Build history of the part. All positions in model axes, mm. A direction names the side the tool comes from. Round coordinates to 2 decimals unless told otherwise and drop trailing zeros. Write each loop counter-clockwise with the first axis right and the second up, starting at its lowest first coordinate (ties: lowest second). Pieces come first, ordered by that corner, then holes.
1) Which spindle directions (+Z, -Z, +X, -X, +Y, -Y) get a long thin tool onto all of the face, cutting with end or side? Do faces 4 (the flat face through (-8, -41, -69.596)), 5 (the cylindrical face through (-1.1, -33.14, -73.57)), 6 (the flat face through (-57.29, -28, -66)). Say none if no direction does.
2) Wall check: probe 1 along X at (y, z) = (-38.1, -51.65); probe 2 along X at (y, z) = (-29, -64); probe 3 along X at (y, z) = (-47, -63). Give the ranges that are in metal, low to high.
3) Saw through at D-D (x = -70). Write the cut outline in (y, z), plus the area to 3 significant figures.
4) Saw through at A-A (z = -73.5). Write the cut outline in (x, y) (1 decimal), plus the area to 3 significant figures.
5) Saw through at B-B (x = 30). Write the cut outline in (y, z).
6) Saw through at C-C (z = -63.5). State how many separate pieces and enclosed holes the cut face has, plus the area to 3 significant figures.
7) Flat gauge pins, fed straight in: pin 1 (12 mm diameter, centred on x = 35.5, z = -64, fed in from -Y); pin 2 (10 mm diameter, centred on y = -45, z = -72, fed in from +X); pin 3 (5 mm diameter, centred on y = -26, z = -71.5, fed in from -X); pin 4 (3 mm diameter, centred on x = 30, z = -63.5, fed in from +Y). Where does each tip first touch, or does it go through?
8) Pull direction Z, two halves, no side cores. Call faces 1 (the cylindrical face through (20.071, -17.413, -63.322)), 2 (the flat face through (67, -41, -52.2)), 3 (the flat face through (0, -46, -70.866)): +Z half, -Z half, draft (parallel to the pull), parting line (faces both ways), or undercut.
Autodesk Inventor part; units mm, degrees
ref_plane "YZ Plane" through (0, 0, 0) normal (1, 0, 0) x (0, 1, 0)
ref_plane "XZ Plane" through (0, 0, 0) normal (0, 1, 0) x (-1, 0, 0)
ref_plane "XY Plane" through (0, 0, 0) normal (0, 0, 1) x (1, 0, 0)
ref_plane "Work Plane1" through (0, 0, -76.2) normal (0, 0, 1) x (1, 0, 0)
sketch "Sketch1" plane through (0, 0, -76.2) normal (0, 0, 1) x (1, 0, 0)
  line L0 (-80, -10.16) -> (80, -10.16)
  circle A0 centre (70, -38.1) radius 4
  circle A1 centre (-70, -38.1) radius 4
  arc A2 (82.7105, -38.1) -> (57.2895, -38.1) centre (70, -38.1) ccw
  arc A3 (57.2895, -38.1) -> (82.4735, -35.6569) centre (70, -38.1) ccw
  arc A4 (-82.4735, -35.6569) -> (-57.2895, -38.1) centre (-70, -38.1) ccw
  line L1 (82.7105, -38.1) -> (80, -10.16)
  line L2 (-82.7105, -38.1) -> (-80, -10.16)
  circle A5 centre (0, -38.1) radius 5.08
  line L3 (17.78, -25.4) -> (17.78, -50.8)
  line L4 (17.78, -50.8) -> (-17.78, -50.8)
  line L5 (-17.78, -50.8) -> (-17.78, -25.4)
  line L6 (-17.78, -25.4) -> (17.78, -50.8) construction
  line L7 (17.78, -25.4) -> (-17.78, -50.8) construction
  line L8 (80, -10.16) -> (-80, -10.16)
  line L9 (-17.78, -15.24) -> (-57.2895, -15.24)
  line L10 (17.78, -15.24) -> (57.2895, -15.24)
  line L11 (57.2895, -38.1) -> (57.2895, -15.24)
  line L12 (-57.2895, -38.1) -> (-57.2895, -15.24)
  line L13 (-17.78, -38.1) -> (-17.78, -15.24)
  line L14 (17.78, -38.1) -> (17.78, -15.24)
  point P0 (0, 0)
  dimension "d0" = 10.16
  dimension "d2" = 35.56
  dimension "d3" = 25.4
extrude "Extrusion1" add sketch "Sketch1" along normal blind 25.4 contours L0 L1 A2 L11 L10 L14 L3 L4 L5 L13 L9 L12 A4 L2 | L1 A3 A2 | A2 L1
sketch "Sketch2" plane through (0, 0, -76.2) normal (0, 0, -1) x (-1, 0, 0)
  circle A0 centre (-70, -38.1) radius 4
  circle A1 centre (-70, -38.1) radius 7.5
  circle A2 centre (70, -38.1) radius 4
  circle A3 centre (70, -38.1) radius 7.5
  point P0 (0, 0)
  dimension "d7" = 15
  dimension "d8" = 15
extrude "Extrusion2" cut sketch "Sketch2" against normal blind 24
sketch "Sketch3" plane through (-17.78, -50.8, -76.2) normal (0, -1, 0) x (1, 0, 0)
  line L0 (0, 0) -> (35.56, 0)
  line L1 (0, 0) -> (0, 25.4)
  line L2 (0, 25.4) -> (35.56, 25.4)
  line L3 (35.56, 0) -> (35.56, 25.4)
  line L4 (12.7, 0) -> (12.7, 25.4)
  line L5 (22.86, 0) -> (22.86, 25.4)
  line L6 (12.7, 25.4) -> (22.86, 25.4)
  line L7 (17.78, 25.4) -> (17.78, 20.32)
  line L8 (22.86, 20.32) -> (12.7, 20.32)
  line L9 (12.7, 20.32) -> (12.7, 10.16)
  line L10 (12.7, 10.16) -> (22.86, 10.16)
  line L11 (22.86, 10.16) -> (22.86, 20.32)
  line L12 (17.78, 10.16) -> (28.575, 10.16)
  line L13 (28.575, 10.16) -> (6.985, 10.16)
  line L14 (28.575, 10.16) -> (6.985, 10.16)
  line L15 (6.985, 10.16) -> (6.985, 6.604)
  line L16 (6.985, 6.604) -> (28.575, 6.604)
  line L17 (28.575, 6.604) -> (28.575, 10.16)
  line L18 (12.7, 5.334) -> (22.86, 5.334)
  line L19 (22.86, 5.334) -> (22.86, 7.874)
  line L20 (22.86, 7.874) -> (12.7, 7.874)
  line L21 (12.7, 7.874) -> (12.7, 5.334)
  line L22 (12.7, 5.334) -> (22.86, 7.874) construction
  line L23 (22.86, 5.334) -> (12.7, 7.874) construction
  point P0 (17.78, 76.2)
  point P1 (17.78, 6.604)
  dimension "d11" = 5.08
  dimension "d12" = 10.16
  dimension "d13" = 10.16
  dimension "d14" = 10.795
  dimension "d15" = 21.59
  dimension "d16" = 21.59
  dimension "d17" = 3.556
  dimension "d18" = 10.16
  dimension "d19" = 2.54
extrude "Extrusion3" cut sketch "Sketch3" against normal blind 21.59 contours L4 L16 L5 L18 | L16 L15 L13 L4 | L4 L20 L5 L16 | L8 L5 L10 L4 | L5 L12 L17 L16 | L4 L10 L5 L20
fillet "Fillet1" radius 10.795 2 edges at (-10.795, -29.21, -67.818) (10.795, -29.21, -67.818)
sketch "Sketch4" plane through (17.78, -15.24, -76.2) normal (0, -1, 0) x (1, 0, 0)
  line L0 (0, 0) -> (39.5095, 0)
  line L1 (0, 25.4) -> (39.5095, 25.4)
  line L2 (-75.0695, 0) -> (-35.56, 0)
  line L3 (62.22, 25.4) -> (-97.78, 25.4)
  line L4 (-97.78, -170.15) -> (-97.78, 69.85)
  line L5 (62.22, -170.15) -> (-97.78, -170.15)
  line L6 (62.22, 69.85) -> (62.22, -170.15)
  line L7 (-97.78, 69.85) -> (62.22, 69.85)
  line L8 (62.22, 0) -> (62.22, 25.4)
  line L9 (62.22, 12.7) -> (32.22, 12.7)
  line L10 (32.22, 12.7) -> (12.22, 12.7)
  circle A0 centre (32.22, 12.7) radius 2
  circle A1 centre (12.22, 12.7) radius 2
  line L11 (62.22, 0) -> (-97.78, 0)
  line L12 (-17.78, 0) -> (-17.78, 2.4889)
  circle A2 centre (-67.78, 12.7) radius 2
  circle A3 centre (-47.78, 12.7) radius 2
  point P0 (-17.78, 76.2)
  dimension "d23" = 30
  dimension "d24" = 20
  dimension "d25" = 4
  dimension "d26" = 4
extrude "Extrusion4" cut sketch "Sketch4" against normal blind 25.4 contours A1 | A0 L10 L9 | L9 L10 A0 | A2 | A3
chamfer "Chamfer1" distance 3.175 angle 45 2 edges at (57.2895, -15.24, -63.5) (-57.2895, -15.24, -63.5)
fillet "Fillet2" radius 7.62 2 edges at (17.78, -15.24, -63.5) (-17.78, -15.24, -63.5)
sketch "Sketch5" plane through (0, 0, -76.2) normal (0, 0, -1) x (-1, 0, 0)
  point P0 (0, 0)
sketch "Sketch6" plane through (0, 0, -50.8) normal (0, 0, 1) x (1, 0, 0)
  line L0 (-57.2895, -18.415) -> (-54.1145, -15.24)
  line L1 (-57.2895, -38.1) -> (-57.2895, -18.415)
  line L2 (-57.2895, -38.1) -> (-22.1843, -15.24)
  line L3 (-54.1145, -15.24) -> (-22.1843, -15.24)
  line L4 (57.2895, -18.415) -> (57.2895, -38.1)
  line L5 (54.1145, -15.24) -> (57.2895, -18.415)
  line L6 (22.1843, -15.24) -> (54.1145, -15.24)
  line L7 (22.1843, -15.24) -> (57.2895, -38.1)
  point P0 (0, 0)
extrude "Extrusion5" add sketch "Sketch6" against normal blind 5.08
properties part number "Bed Slide"
Evaluation:
1. face 4: -Y
1. face 5: +Z, -Z
1. face 6: -Z, -Y
2. probe 1: x = -82.71 to -74, -66 to -57.29, -17.78 to -5.08, 5.08 to 17.78, 57.29 to 66, 74 to 82.71
2. probe 2: x = -81.83 to -57.29, -17.78 to 17.78, 57.29 to 81.83
2. probe 3: x = -79.07 to -60.93, -17.78 to -5.08, 5.08 to 17.78, 60.93 to 79.07
3. outline: (-50.81, -76.2) - (-45.6, -76.2) - (-45.6, -52.2) - (-42.1, -52.2) - (-42.1, -50.8) - (-50.81, -50.8) - close; (-34.1, -52.2) - (-30.6, -52.2) - (-30.6, -76.2) - (-10.16, -76.2) - (-10.16, -50.8) - (-34.1, -50.8) - close
3. area: 661 mm2
4. outline: (-82.7, -38.1) arc R12.7 ccw to (-57.3, -38.1) - (-57.3, -18.4) - (-54.1, -15.2) - (-25.4, -15.2) arc R7.6 cw to (-17.8, -22.9) - (-17.8, -50.8) - (17.8, -50.8) - (17.8, -22.9) arc R7.6 cw to (25.4, -15.2) - (54.1, -15.2) - (57.3, -18.4) - (57.3, -38.1) arc R12.7 ccw to (82.7, -38.1) arc R12.7 ccw to (82.5, -35.7) - (80, -10.2) - (-80, -10.2) - close; hole circle Ø15 at (-70, -38.1); hole circle Ø10.2 at (0, -38.1); hole circle Ø15 at (70, -38.1)
4. area: 3,300 mm2
5. outline: (-20.33, -55.88) - (-15.24, -55.88) - (-15.24, -61.5) - (-10.16, -61.5) - (-10.16, -50.8) - (-20.33, -50.8) - close; (-15.24, -76.2) - (-10.16, -76.2) - (-10.16, -65.5) - (-15.24, -65.5) - close
6. separate pieces: 5
6. enclosed holes: 2
6. area: 3,080 mm2
7. pin 1: stops at y = -15.24
7. pin 2: stops at x = 82.57
7. pin 3: stops at x = -81.78
7. pin 4: passes through
8. face 1: draft
8. face 2: -Z half
8. face 3: undercut
